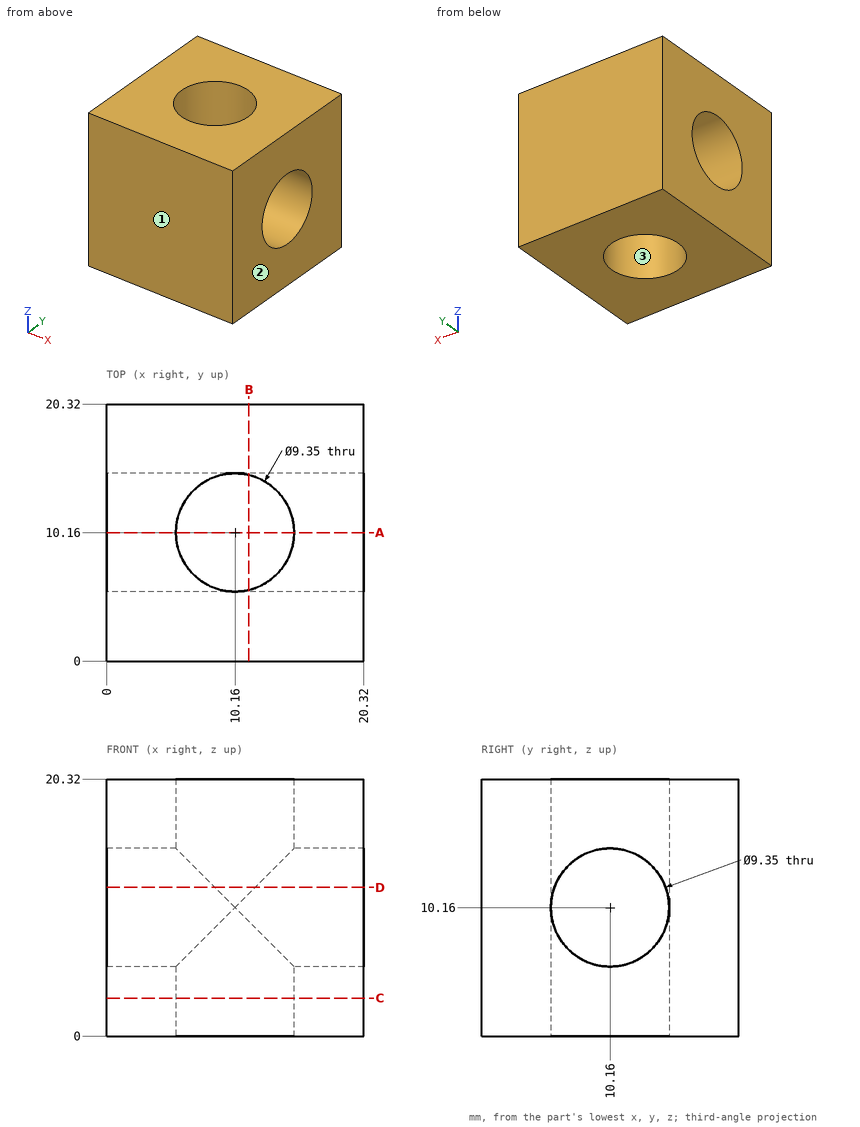
Study the drawing (mm; zero at the part's minimum x, y, z) and answer. Round coordinates to 2 decimals unless told otherwise and drop trailing zeros. Order: outer loops, then holes, each group sorted by start corner. A loop starts at its lowest first (then second) coordinate and runs counter-clockwise, first axis right, second up. Notation, with made-up numbers: (88, -10.5) -> (136, -10.5) arc R9 cw to (136, -3.5) -> close; hole circle Ø6 at (76, 2). An arc over 180 degrees is marked (long way). Answer as CSV lines item,"result". Start each with the question number.
(1) The part is cut by section C-C (z = 3). Determine the outline of the cut face in (x, y) (3 decimals).
(2) The part is cut by section D-D (z = 11.75). Determine the outline of the cut face in (x, y) (3 decimals).
(3) Find the intervals of material crossed by probe 1 along Y at (x, z) = (10.16, 3) (3 decimals); probe 2 along X at (y, z) = (10, 16.5), in increasing order. Write a range as from..to.
(4) The part is cut by section B-B (x = 11.25). Determine the outline of the cut face in (y, z) (3 decimals), then the cut area to 3 significant figures.
(5) For a pull along Y with two mould halves and no side action, classify the marked faces 1, 2 and 3 as +Y half, -Y half, draft (parallel to the pull), parting line (faces both ways), or undercut.
(6) The part is cut by section A-A (y = 10.16). Determine the outline of the cut face in (x, z) (3 decimals), then the cut area to 3 significant figures.
Evaluation:
1,outline,"(0, 0) -> (20.32, 0) -> (20.32, 20.32) -> (0, 20.32) -> close; hole circle Ø9.35 at (10.16, 10.16)"
2,outline,"(0, 0) -> (20.32, 0) -> (20.32, 5.764) -> (11.75, 5.764) arc R4.675 cw to (8.57, 5.764) -> (0, 5.764) -> close; (0, 14.556) -> (8.57, 14.556) arc R4.675 cw to (11.75, 14.556) -> (20.32, 14.556) -> (20.32, 20.32) -> (0, 20.32) -> close"
3,probe 1,"0..5.485, 14.835..20.32"
3,probe 2,"0..5.49, 14.83..20.32"
4,outline,"(0, 0) -> (5.614, 0) -> (5.614, 9.07) arc R4.675 cw to (5.614, 11.25) -> (5.614, 20.32) -> (0, 20.32) -> close; (14.706, 0) -> (20.32, 0) -> (20.32, 20.32) -> (14.706, 20.32) -> (14.706, 11.25) arc R4.675 cw to (14.706, 9.07) -> close"
4,area,"228 mm²"
5,face 1,"-Y half"
5,face 2,"draft"
5,face 3,"undercut"
6,outline,"(0, 0) -> (5.485, 0) -> (5.485, 5.485) -> (0, 5.485) -> close; (0, 14.835) -> (5.485, 14.835) -> (5.485, 20.32) -> (0, 20.32) -> close; (14.835, 0) -> (20.32, 0) -> (20.32, 5.485) -> (14.835, 5.485) -> close; (14.835, 14.835) -> (20.32, 14.835) -> (20.32, 20.32) -> (14.835, 20.32) -> close"
6,area,"120 mm²"
